Verification items for the finished model (mm, model axes). A direction names the side the tool comes from. Coordinates: 2 decimals unless noted, no trailing zeros. Order: outer loops, then holes, each group sorted by start corner. A loop starts at its lowest first (then second) coordinate and runs counter-clockwise, first axis right, second up. Notation, with made-up numbers: M 29,-9.75 L 57,-9.75 A14 ccw 57,14.25 Z; hole C -8,-20.75 d5. An arc over 180 degrees is marked long. Write item = value, one per line.
Autodesk Inventor part; units mm, degrees
ref_plane "YZ Plane" through (0, 0, 0) normal (1, 0, 0) x (0, 1, 0)
ref_plane "XZ Plane" through (0, 0, 0) normal (0, 1, 0) x (-1, 0, 0)
ref_plane "XY Plane" through (0, 0, 0) normal (0, 0, 1) x (1, 0, 0)
sketch "Sketch1" plane through (0, 0, 0) normal (0, 0, 1) x (1, 0, 0)
  line L0 (0, 0) -> (0, 38.1)
  line L1 (0, 38.1) -> (-12.7, 38.1)
  line L2 (-12.7, 38.1) -> (-12.7, 0)
  line L3 (-12.7, 0) -> (0, 0)
  dimension "d0" = 38.1
  dimension "d1" = 12.7
extrude "Extrusion1" add sketch "Sketch1" along normal blind 6.35
sketch "Sketch2" plane through (0, 0, 6.35) normal (0, 0, 1) x (1, 0, 0)
  line L0 (0, 38.1) -> (-12.7, 38.1)
  line L1 (-12.7, 38.1) -> (-12.7, 0)
  line L2 (-12.7, 0) -> (0, 0)
  line L3 (0, 0) -> (0, 38.1)
  line L4 (-6.35, 38.1) -> (-6.35, 0) construction
  line L5 (-6.35, 38.1) -> (-6.35, 33.02)
  circle A0 centre (-6.35, 33.02) radius 2.413
  line L6 (-6.35, 33.02) -> (-6.35, 24.257)
  circle A1 centre (-6.35, 24.257) radius 2.413
  dimension "d4" = 5.08
  dimension "d5" = 4.826
  dimension "d6" = 8.763
  dimension "d7" = 4.826
extrude "Extrusion2" cut sketch "Sketch2" against normal up to next contours A1 | A0 L6 L5 | L5 L6 A0
sketch "Sketch3" plane through (-12.7, 0, 0) normal (0, -1, 0) x (1, 0, 0)
  line L0 (0, 0) -> (12.7, 0)
  line L1 (12.7, 0) -> (12.7, 6.35)
  line L2 (0, 6.35) -> (12.7, 6.35)
  line L3 (0, 0) -> (0, 6.35)
  line L4 (0, 3.175) -> (12.7, 3.175) construction
  line L5 (6.35, 6.35) -> (6.35, 0) construction
  line L6 (-19.05, -22.225) -> (-19.05, 28.575)
  line L7 (-19.05, 28.575) -> (31.75, 28.575)
  line L8 (31.75, 28.575) -> (31.75, -22.225)
  line L9 (31.75, -22.225) -> (-19.05, -22.225)
  line L10 (-19.05, -22.225) -> (31.75, 28.575) construction
  line L11 (-19.05, 28.575) -> (31.75, -22.225) construction
  point P0 (6.35, 3.175)
  dimension "d10" = 50.8
  dimension "d11" = 50.8
extrude "Extrusion3" add sketch "Sketch3" against normal blind 6.35
sketch "Sketch4" plane through (-31.75, 0, 28.575) normal (0, -1, 0) x (1, 0, 0)
  line L0 (50.8, -50.8) -> (50.8, 0)
  line L1 (50.8, 0) -> (0, 0)
  line L2 (0, 0) -> (0, -50.8)
  line L3 (0, -50.8) -> (50.8, -50.8)
  line L4 (0, -25.4) -> (50.8, -25.4) construction
  line L5 (0, -25.4) -> (0, -13.208)
  line L6 (0, -13.208) -> (5.08, -13.208)
  line L7 (5.08, -13.208) -> (25.4, -13.208) construction
  line L8 (5.08, -14.5288) -> (25.4, -14.5288)
  line L9 (25.4, -11.8872) -> (5.08, -11.8872)
  arc A0 (5.08, -11.8872) -> (5.08, -14.5288) centre (5.08, -13.208) ccw
  arc A1 (25.4, -14.5288) -> (25.4, -11.8872) centre (25.4, -13.208) ccw
  line L10 (5.08, -36.2712) -> (25.4, -36.2712)
  line L11 (25.4, -38.9128) -> (5.08, -38.9128)
  arc A2 (5.08, -36.2712) -> (5.08, -38.9128) centre (5.08, -37.592) ccw
  arc A3 (25.4, -38.9128) -> (25.4, -36.2712) centre (25.4, -37.592) ccw
  point P0 (31.75, -28.575)
  point P1 (15.24, -13.208)
  dimension "d14" = 12.192
  dimension "d16" = 5.08
  dimension "d17" = 20.32
  dimension "d18" = 2.6416
extrude "Extrusion4" cut sketch "Sketch4" against normal blind 6.35 contours A0 L9 A1 L8 | L10 A3 L11 A2
sketch "Sketch6" plane through (-31.75, 0, 28.575) normal (0, -1, 0) x (1, 0, 0)
  line L0 (25.4, -14.5288) -> (5.08, -14.5288)
  arc A0 (5.08, -11.8872) -> (5.08, -14.5288) centre (5.08, -13.208) ccw
  line L1 (5.08, -11.8872) -> (25.4, -11.8872)
  arc A1 (25.4, -14.5288) -> (25.4, -11.8872) centre (25.4, -13.208) ccw
  arc A2 (5.08, -36.2712) -> (5.08, -38.9128) centre (5.08, -37.592) ccw
  line L2 (5.08, -36.2712) -> (25.4, -36.2712)
  arc A3 (25.4, -38.9128) -> (25.4, -36.2712) centre (25.4, -37.592) ccw
  line L3 (25.4, -38.9128) -> (5.08, -38.9128)
  line L4 (50.8, -50.8) -> (50.8, 0)
  line L5 (50.8, 0) -> (0, 0)
  line L6 (0, 0) -> (0, -50.8)
  line L7 (0, -50.8) -> (50.8, -50.8)
  line L8 (26.7208, -13.208) -> (26.7208, -50.8)
  line L9 (26.7208, -13.208) -> (26.7208, 0)
  line L10 (26.7208, 0) -> (26.7208, 17.78)
  line L11 (26.7208, -50.8) -> (26.7208, -68.58)
  line L12 (26.7208, 17.78) -> (50.8, 17.78)
  line L13 (50.8, 17.78) -> (50.8, 0)
  line L14 (26.7208, -68.58) -> (50.8, -68.58)
  line L15 (50.8, -68.58) -> (50.8, -50.8)
  point P0 (31.75, -28.575)
  dimension "d23" = 17.78
  dimension "d24" = 17.78
extrude "Extrusion5" add sketch "Sketch6" against normal blind 6.35 contours L10 L12 L13 L5 | L7 L15 L14 L11
sketch "Sketch7" plane through (-31.75, 0, -22.225) normal (0, -1, 0) x (1, 0, 0)
  line L0 (25.4, 36.2712) -> (5.08, 36.2712)
  arc A0 (5.08, 38.9128) -> (5.08, 36.2712) centre (5.08, 37.592) ccw
  line L1 (5.08, 38.9128) -> (25.4, 38.9128)
  arc A1 (25.4, 36.2712) -> (25.4, 38.9128) centre (25.4, 37.592) ccw
  arc A2 (5.08, 14.5288) -> (5.08, 11.8872) centre (5.08, 13.208) ccw
  line L2 (5.08, 14.5288) -> (25.4, 14.5288)
  arc A3 (25.4, 11.8872) -> (25.4, 14.5288) centre (25.4, 13.208) ccw
  line L3 (25.4, 11.8872) -> (5.08, 11.8872)
  line L4 (50.8, -17.78) -> (50.8, 68.58)
  line L5 (50.8, 68.58) -> (26.7208, 68.58)
  line L6 (26.7208, 68.58) -> (26.7208, 50.8)
  line L7 (26.7208, 50.8) -> (0, 50.8)
  line L8 (0, 50.8) -> (0, 0)
  line L9 (0, 0) -> (26.7208, 0)
  line L10 (26.7208, 0) -> (26.7208, -17.78)
  line L11 (26.7208, -17.78) -> (50.8, -17.78)
  line L12 (25.4, 37.592) -> (25.4, 13.208) construction
  line L13 (25.4, 25.4) -> (50.8, 25.4) construction
  line L14 (38.1, -7.62) -> (38.1, 58.42) construction
  line L15 (39.4335, -7.62) -> (39.4335, 58.42)
  line L16 (36.7665, 58.42) -> (36.7665, -7.62)
  arc A4 (36.7665, -7.62) -> (39.4335, -7.62) centre (38.1, -7.62) ccw
  arc A5 (39.4335, 58.42) -> (36.7665, 58.42) centre (38.1, 58.42) ccw
  point P0 (31.75, 22.225)
  point P1 (38.1, 25.4)
  dimension "d27" = 33.02
  dimension "d28" = 2.667
extrude "Extrusion6" cut sketch "Sketch7" against normal blind 6.35 contours A4 L16 A5 L15
sketch "Sketch8" plane through (-31.75, 0, -22.225) normal (0, -1, 0) x (1, 0, 0)
  line L0 (0, 0) -> (0, 50.8)
  line L1 (0, 0) -> (-6.9749, 6.5838)
  line L2 (-6.9749, 6.5838) -> (0, 10.4686)
  line L3 (0, 10.4686) -> (-6.3127, 15.1611)
  line L4 (-6.3127, 15.1611) -> (0, 20.9868)
  line L5 (-5.6991, 27.1623) -> (0, 31.5381)
  line L6 (0, 20.9868) -> (-5.6991, 27.1623)
  line L7 (0, 31.5381) -> (-5.7764, 35.832)
  line L8 (-5.7764, 35.832) -> (0, 39.0492)
  line L9 (-5.4281, 43.0842) -> (0, 39.0492)
  line L10 (-5.7764, 43.343) -> (0, 46.5602)
  line L11 (-5.7036, 50.8) -> (0, 50.8)
  line L12 (0, 50.8) -> (0, 46.5602)
  line L13 (-5.7036, 50.8) -> (0, 46.5602)
  line L14 (-5.7764, 43.343) -> (0, 39.0492)
  point P0 (31.75, 22.225)
  point P1 (-5.4281, 43.0842)
extrude "Extrusion7" add sketch "Sketch8" against normal blind 6.35
fillet "Fillet1" radius 1.27 1 edges at (-38.7249, 3.175, -15.6412)
fillet "Fillet2" radius 1.27 1 edges at (-38.0627, 3.175, -7.0639)
fillet "Fillet3" radius 1.27 4 edges at (-37.4491, 3.175, 4.9373) (-37.5264, 3.175, 13.607) (-37.5264, 3.175, 21.118) (-37.4536, 3.175, 28.575)
sketch "Sketch9" plane through (-5.0292, 0, -40.005) normal (0, -1, 0) x (1, 0, 0)
  line L0 (-26.7208, 17.78) -> (0, 17.78)
  line L1 (-7.995, 17.78) -> (-7.995, 5.2737)
  line L2 (-20.7092, 17.78) -> (-20.7092, 5.4549)
  arc A0 (-20.7092, 5.4549) -> (-7.995, 2.5659) centre (-13.3604, 8.3747) ccw
  line L3 (-7.995, 5.2737) -> (-7.995, 2.5659)
  line L4 (24.0792, 0) -> (24.0792, 86.36)
  line L5 (24.0792, 43.18) -> (-30.9425, 43.18) construction
  line L6 (-28.5871, 68.58) -> (0, 68.58)
  line L7 (-7.995, 68.58) -> (-7.995, 82.6845)
  line L8 (-20.7092, 68.58) -> (-20.7092, 82.6845)
  line L9 (-20.7092, 82.6845) -> (-20.7092, 87.4507)
  line L10 (-7.995, 82.6845) -> (-7.995, 87.6044)
  arc A1 (-7.995, 87.6044) -> (-20.7092, 87.4507) centre (-14.2936, 82.6845) ccw
  point P0 (5.0292, 40.005)
extrude "Extrusion8" add sketch "Sketch9" against normal blind 6.35
properties part number "camera_cutout"
Item 1: Scan lines: L1, parallel to Y at x = -6.35, z = 4.5; L2, parallel to Z at x = -10, y = 5.5 (3 decimals); L3, parallel to Z at x = -19, y = 5.5. Record each from-to range of solid material in increasing order. Write a range as from..to.
Report:
L1 = 0..21.84, 26.67..30.61, 35.43..38.1
L2 = -22.225..-10.338, -7.696..14.046, 16.688..28.575
L3 = -39.51..-10.34, -7.7..14.05, 16.69..50.67
Item 2: Sectioned sample at B-B, the plane y = 33.02. Enter the section's corners in (x, z), then the cut area to 3 significant figures.
Report:
outline = M -12.7,0 L -8.76,0 L -8.76,6.35 L -12.7,6.35 Z; M -3.94,0 L 0,0 L 0,6.35 L -3.94,6.35 Z
area = 50.0 mm^2
Item 3: Gauge pin test, flat ends, axial feed: pin 1 (10 mm diameter, centred on y = 25.5, z = 14, fed in from +X); pin 2 (7 mm diameter, centred on x = -18, y = 4.5, fed in from -Z); pin 3 (1.9 mm diameter, centred on y = 2.5, z = 39, fed in from -X); pin 4 (6.5 mm diameter, centred on x = -28.5, y = 3, fed in from -Z). Record the tip position at first contact, or that the pin passes through.
Report:
pin_1 = through
pin_2 = -39.54
pin_3 = -25.74
pin_4 = -35.56
Item 4: Sectioned sample at D-D, the plane y = 12.5. Enter the section's corners in (x, z), then the cut area to 3 significant figures.
Report:
outline = M -12.7,0 L 0,0 L 0,6.35 L -12.7,6.35 Z
area = 80.6 mm^2
Item 5: Tool access check on faces 5 (the flat face through (-13.024, 3, 38)), 6 (the flat face through (-34.52, 3.13, -13.3)), 7 (the flat face through (-5.029, 3, -31)), 8 (the flat face through (-29, 3, -22.225)), 9 (the cylindrical face through (6.32, 3.13, -31.18)). Record the directions out of +Z, -Z, +X, -X, +Y, -Y that give a thin tool (end or side, any length) a straight path to the whole face; none if there is none.
Report:
face_5 = +Z, +Y, -Y
face_6 = -X, +Y, -Y
face_7 = -Z, +Y, -Y
face_8 = -Z, -X, +Y, -Y
face_9 = +Y, -Y
Item 6: Sectioned sample at C-C, the plane z = 1.5. Enter the section's corners in (x, y), then the cut area to 3 significant figures.
Report:
outline = M -34.28,0 L 5.02,0 L 5.02,6.35 L 0,6.35 L 0,38.1 L -12.7,38.1 L -12.7,6.35 L -34.28,6.35 Z; M 7.68,0 L 19.05,0 L 19.05,6.35 L 7.68,6.35 Z; hole C -6.35,24.26 d4.83; hole C -6.35,33.02 d4.83
area = 688 mm^2
Item 7: Release check for a two-part mould opening along Z. For faces 1 (the flat face through (-9, 3, 28.575)), 2 (the flat face through (-34.567, 3.131, -19.566)), 3 (the flat face through (-34.08, 3.131, 7.524)), 4 (the flat face through (-13.024, 3, -30)) record: pulls with the +Z half, pulls with the -Z half, needs draft (parallel to the pull), parting line crosses it, or undercut.
Report:
face_1 = pulls with the +Z half
face_2 = pulls with the -Z half
face_3 = undercut
face_4 = needs draft
